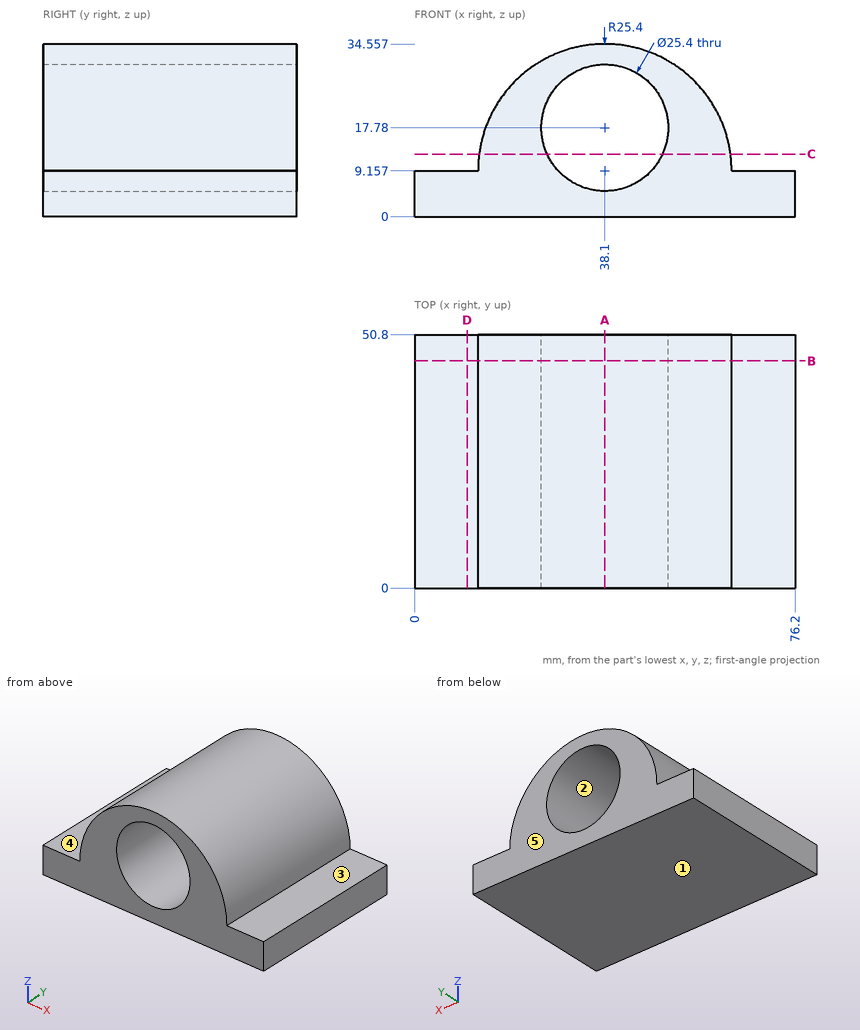
Print and shaded views of the part. All mm, measured from the part's lowest x, y and z. A direction names the side the tool comes from. Give positions to 0.01 mm unless a question says otherwise; leave off trailing zeros. Write each loop counter-clockwise with the first axis right and the second up, starting at its lowest first coordinate (ties: lowest second). Pieces come first, ordered by that corner, then holes. Notation, with made-up numbers: (46.25, 38.5) -> (102.25, 38.5) arc R9 ccw to (102.25, 50.5) -> close; hole circle Ø10 at (-34.75, 17). An arc over 180 degrees is marked (long way). Write each question's results on one line, items separated by ' | '.
1. Cut at A-A, the plane x = 38.1. Write the cut outline in (y, z), then the cut area to 3 significant figures.
Geometry check:
outline: (0, 0) -> (50.8, 0) -> (50.8, 5.08) -> (0, 5.08) -> close; (0, 30.48) -> (50.8, 30.48) -> (50.8, 34.56) -> (0, 34.56) -> close | area: 465 mm²
2. Two-plate mould, pull along Z, no slides. Class the marked faces 1, 2 and 3: pulls with the +Z half, pulls with the -Z half, needs draft (parallel to the pull), parting line crosses it, or undercut.
Geometry check:
face 1: pulls with the -Z half | face 2: undercut | face 3: pulls with the +Z half
3. Cut at C-C, the plane z = 12.5. Write the cut outline in (x, y), then the cut area to 3 significant figures.
Geometry check:
outline: (12.92, 0) -> (26.55, 0) -> (26.55, 50.8) -> (12.92, 50.8) -> close; (49.65, 0) -> (63.28, 0) -> (63.28, 50.8) -> (49.65, 50.8) -> close | area: 1,380 mm²
4. Cut at D-D, the plane x = 10.5. Write the cut outline in (y, z), then the cut area to 3 significant figures.
Geometry check:
outline: (0, 0) -> (50.8, 0) -> (50.8, 9.16) -> (0, 9.16) -> close | area: 465 mm²
5. Cut at B-B, the plane y = 45.5. Write the cut outline in (x, z).
Geometry check:
outline: (0, 0) -> (76.2, 0) -> (76.2, 9.16) -> (63.5, 9.16) arc R25.4 ccw to (12.7, 9.16) -> (0, 9.16) -> close; hole circle Ø25.4 at (38.1, 17.78)
6. Wall check: probe 1 along Z at (x, y) = (38, 31); probe 2 along Z at (x, y) = (72.5, 13); probe 3 along X at (y, z) = (29, 28). Give the ranges that are in metal, low to high. Write a range as [from, to].
Geometry check:
probe 1: [0, 5.08], [30.48, 34.56] | probe 2: [0, 9.16] | probe 3: [21.07, 30.56], [45.64, 55.13]
7. Which spindle directions (+Z, -Z, +X, -X, +Y, -Y) get a long thin tool onto all of the face, cutting with end or side? Do the marked faces 4 and 5. Say none if no direction does.
Geometry check:
face 4: +Z, -X, +Y, -Y | face 5: +Z, -Z, +X, -X, +Y
8. Drop flat-ended pins along their axis: P1, Ø5, axis at y = 35, z = 28, coming from the +X side; P2, Ø6, axis at x = 60.5, z = 30.5, coming from the +Y side; P3, Ø12, axis at y = 32.5, z = 31, coming from the +X side; P4, Ø1, axis at x = 8, y = 10, coming from the +Z side. Give the stop position or say it passes through.
Geometry check:
P1: x = 57.54 | P2: through | P3: x = 57.95 | P4: z = 9.16
